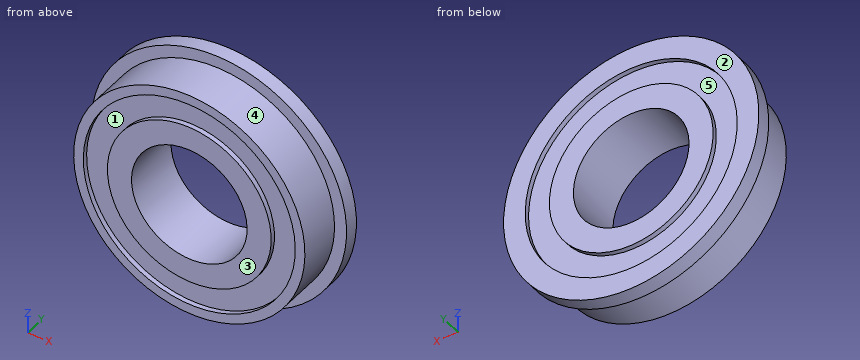
```python
from build123d import *

# Parameters (mm, degrees)
SKETCH1_R           = 12
SKETCH1_R_2         = 6
BOSS_EXTRUDE1_DEPTH = 6
SKETCH1_3_R         = 13.25
SKETCH1_3_R_2       = 12
BOSS_EXTRUDE2_DEPTH = 1.5
SKETCH2_R           = 11
SKETCH2_R_2         = 8.5
CUT_EXTRUDE1_DEPTH  = 0.5
CUT_EXTRUDE2_START  = -0.5
SKETCH3_R           = 11
SKETCH3_R_2         = 8.5
CUT_EXTRUDE2_DEPTH  = 0.5


with BuildPart() as part:
    # Sketch1 → Boss-Extrude1 (new body)
    with BuildSketch(Plane(origin=(0, 0, 0), x_dir=(1, 0, 0), z_dir=(0, 1, 0))):
        with Locations(Location((0, 0, 0), (0, 0, 270))):
            Circle(SKETCH1_R)
        with Locations(Location((0, 0, 0), (0, 0, 270))):
            Circle(SKETCH1_R_2, mode=Mode.SUBTRACT)
    extrude(amount=-BOSS_EXTRUDE1_DEPTH)

    # Sketch1_3 → Boss-Extrude2 (add)
    with BuildSketch(Plane(origin=(0, 0, 0), x_dir=(1, 0, 0), z_dir=(0, 1, 0))):
        with Locations(Location((0, 0, 0), (0, 0, 270))):
            Circle(SKETCH1_3_R)
        with Locations(Location((0, 0, 0), (0, 0, 270))):
            Circle(SKETCH1_3_R_2, mode=Mode.SUBTRACT)
    extrude(amount=-BOSS_EXTRUDE2_DEPTH)

    # Sketch2 → Cut-Extrude1 (cut)
    with BuildSketch(Plane(origin=(0, 0, 0), x_dir=(1, 0, 0), z_dir=(0, 1, 0))):
        with Locations(Location((0, 0, 0), (0, 0, 270))):
            Circle(SKETCH2_R)
        with Locations(Location((0, 0, 0), (0, 0, 270))):
            Circle(SKETCH2_R_2, mode=Mode.SUBTRACT)
    extrude(amount=-CUT_EXTRUDE1_DEPTH, mode=Mode.SUBTRACT)

    # Sketch3 → Cut-Extrude2 (cut)
    with BuildSketch(Plane.XZ.offset(6).offset(CUT_EXTRUDE2_START)):
        with Locations(Location((0, 0, 0), (0, 0, 90))):
            Circle(SKETCH3_R)
        with Locations(Location((0, 0, 0), (0, 0, 90))):
            Circle(SKETCH3_R_2, mode=Mode.SUBTRACT)
    extrude(amount=CUT_EXTRUDE2_DEPTH, mode=Mode.SUBTRACT)


solid = part.part
```
For this review, take the finished solid that the model builds, in its own axes (mm). Face numbers are marked on the shaded views. A direction names the side the tool comes from. Round coordinates to 2 decimals unless told otherwise and drop trailing zeros. Write each loop counter-clockwise with the first axis right and the second up, starting at its lowest first coordinate (ties: lowest second). Pieces come first, ordered by that corner, then holes. Notation, with made-up numbers: (83, 35) -> (104, 35) arc R27 cw to (104, 55) -> close; hole circle Ø2 at (-26, -35). An arc over 180 degrees is marked (long way). One line per question, with ' | ' between items. Start each with the question number.
(1) Add section C-C, the plane y = -2.45. Write out the cut boundary in (x, z).
(2) For line 1 along X through (y, z) = (-4.55, 0); line 2 along Y through (x, z) = (-9.5, -8.75); line 3 along X through (y, z) = (-3.5, -4), list the stretches that pass through material, from the lowest coordinate up. Write a range as from..to.
(3) Insertion check: P1, Ø3, axis at x = -1.5, z = -4, coming from the +Y side; P2, Ø3, axis at x = 0, z = -5, coming from the -Y side; P3, Ø2, axis at x = 2, y = -2, coming from the -Z side; P4, Ø1, axis at x = 6.5, z = -7, coming from the -Y side. Each pin has a flat end and moves straight along its axis. Give the tip position at first contact, or say it passes through.
(4) Add section D-D, the plane x = -7.25. Write out the cut boundary in (y, z), plus the area to 3 significant figures.
(5) Add section A-A, the plane x = 0. Write out the cut boundary in (y, z), plus the area to 4 significant figures.
(6) Add section B-B, the plane z = 0. Write out the cut boundary in (x, y), plus the area to 4 significant figures.
(7) Mouldability with a two-part tool opening along Z and no side actions: class the marked faces 3, 4 and 5 as released by +Z, released by -Z, zero draft, split by the parting line, or undercut.
(8) Tool access review of the marked faces 1 and 2: name each direction out of +Z, -Z, +X, -X, +Y, -Y from which nothing blocks a thin tool from reaching the whole face with its end or side.
Answer list:
1) outline: circle Ø24 at (0, 0); hole circle Ø12 at (0, 0)
2) line 1: -12..-6, 6..12 | line 2: -1.5..0 | line 3: -11.31..-4.47, 4.47..11.31
3) P1: through | P2: y = -6 | P3: z = -13.2 | P4: y = -5.5
4) outline: (-6, -9.56) -> (-1.5, -9.56) -> (-1.5, -11.09) -> (0, -11.09) -> (0, -8.27) -> (-0.5, -8.27) -> (-0.5, -4.44) -> (0, -4.44) -> (0, 4.44) -> (-0.5, 4.44) -> (-0.5, 8.27) -> (0, 8.27) -> (0, 11.09) -> (-1.5, 11.09) -> (-1.5, 9.56) -> (-6, 9.56) -> (-6, 8.27) -> (-5.5, 8.27) -> (-5.5, 4.44) -> (-6, 4.44) -> (-6, -4.44) -> (-5.5, -4.44) -> (-5.5, -8.27) -> (-6, -8.27) -> close | area: 112 mm²
5) outline: (-6, -12) -> (-1.5, -12) -> (-1.5, -13.25) -> (0, -13.25) -> (0, -11) -> (-0.5, -11) -> (-0.5, -8.5) -> (0, -8.5) -> (0, -6) -> (-6, -6) -> (-6, -8.5) -> (-5.5, -8.5) -> (-5.5, -11) -> (-6, -11) -> close; (-6, 6) -> (0, 6) -> (0, 8.5) -> (-0.5, 8.5) -> (-0.5, 11) -> (0, 11) -> (0, 13.25) -> (-1.5, 13.25) -> (-1.5, 12) -> (-6, 12) -> (-6, 11) -> (-5.5, 11) -> (-5.5, 8.5) -> (-6, 8.5) -> close | area: 70.75 mm²
6) outline: (-13.25, -1.5) -> (-12, -1.5) -> (-12, -6) -> (-11, -6) -> (-11, -5.5) -> (-8.5, -5.5) -> (-8.5, -6) -> (-6, -6) -> (-6, 0) -> (-8.5, 0) -> (-8.5, -0.5) -> (-11, -0.5) -> (-11, 0) -> (-13.25, 0) -> close; (6, -6) -> (8.5, -6) -> (8.5, -5.5) -> (11, -5.5) -> (11, -6) -> (12, -6) -> (12, -1.5) -> (13.25, -1.5) -> (13.25, 0) -> (11, 0) -> (11, -0.5) -> (8.5, -0.5) -> (8.5, 0) -> (6, 0) -> close | area: 70.75 mm²
7) face 3: zero draft | face 4: split by the parting line | face 5: undercut
8) face 1: -Y | face 2: +Z, -Z, +X, -X, +Y
